```python
from build123d import *

# Parameters (mm, degrees)
SKETCH_1_W      = 5
SKETCH_1_H      = 60
EXTRUDE_1_DEPTH = 2
SKETCH_2_W      = 3
SKETCH_2_H      = 10
EXTRUDE_2_DEPTH = 10.5
SKETCH_3_W      = 15
SKETCH_3_H      = 60
EXTRUDE_3_DEPTH = 1.5


with BuildPart() as part:
    # 草图1 → 凸台-拉伸1 (new body)
    with BuildSketch(Plane(origin=(0, 0, 0), x_dir=(0, 0, -1), z_dir=(1, 0, 0))):
        with Locations((-1, 0)):
            Rectangle(SKETCH_1_W, SKETCH_1_H)
    extrude(amount=EXTRUDE_1_DEPTH)

    # 草图2 → 凸台-拉伸2 (add)
    with BuildSketch(Plane.ZY):
        with Locations((0, 20)):
            Rectangle(SKETCH_2_W, SKETCH_2_H)
        Rectangle(SKETCH_2_W, SKETCH_2_H)
        with Locations((0, -20)):
            Rectangle(SKETCH_2_W, SKETCH_2_H)
    extrude(amount=EXTRUDE_2_DEPTH)

    # 草图3 → 凸台-拉伸3 (add)
    with BuildSketch(Plane.ZY.offset(10.5)):
        Rectangle(SKETCH_3_W, SKETCH_3_H)
    extrude(amount=EXTRUDE_3_DEPTH)


solid = part.part
```
Check sheet for the modelled part. Datum: model origin and axes. Units: mm. A direction names the side the tool comes from. Round coordinates to 2 decimals unless told otherwise and drop trailing zeros. Loops run counter-clockwise (first coordinate to the right, second up) from the corner with the lowest first, then second, coordinate; pieces in that order, holes last. Notation, with made-up numbers: M -36,39 L 16,39 A29 cw 16,68 Z; hole C 87,-12.75 d10. An arc over 180 degrees is marked long. Answer as a JSON object with one key per item and string values.
1. Section check A-A (x = -3.5). Record the boundary of the cut face in (y, z), plus the area to 3 significant figures.
Reply:
{"outline": "M -25,-1.5 L -15,-1.5 L -15,1.5 L -25,1.5 Z; M -5,-1.5 L 5,-1.5 L 5,1.5 L -5,1.5 Z; M 15,-1.5 L 25,-1.5 L 25,1.5 L 15,1.5 Z", "area": "90.0 mm²"}
2. Scan lines: line 1 (Y direction, x = -10, z = 1); line 2 (X direction, y = 0, z = 2); line 3 (X direction, y = 3, z = -3.75). Record each from-to range of solid material in increasing order.
Reply:
{"line 1": "y = -25 to -15, -5 to 5, 15 to 25", "line 2": "x = -12 to -10.5, 0 to 2", "line 3": "x = -12 to -10.5"}
3. Access from +Z, -Z, +X, -X, +Y, -Y to the whole of each face (thin tool, end or side, straight path). Record for faces 5 (the flat face through (-5, -25, 0)), 6 (the flat face through (-5, 15, 0)), 7 (the flat face through (1, 0, 3.5)).
Reply:
{"face 5": "+Z, -Z, -Y", "face 6": "+Z, -Z", "face 7": "+Z, +X, +Y, -Y"}
4. Gauge pin test, flat ends, axial feed: P1, Ø6, axis at x = 0, y = 16, coming from the +Z side; P2, Ø4, axis at x = -8, y = -3.5, coming from the -Z side; P3, Ø1.5, axis at x = -6, z = 0, coming from the +Y side. Record the tip position at first contact, or that the pin passes through.
Reply:
{"P1": "stops at z = 3.5", "P2": "stops at z = -1.5", "P3": "stops at y = 25"}
5. Section check B-B (z = 2.25). Record the boundary of the cut face in (x, y).
Reply:
{"outline": "M -12,-30 L -10.5,-30 L -10.5,30 L -12,30 Z; M 0,-30 L 2,-30 L 2,30 L 0,30 Z"}
6. Section check C-C (y = -6.5). Record the boundary of the cut face in (x, z).
Reply:
{"outline": "M -12,-7.5 L -10.5,-7.5 L -10.5,7.5 L -12,7.5 Z; M 0,-1.5 L 2,-1.5 L 2,3.5 L 0,3.5 Z"}
7. Section check D-D (y = 19.5). Record the boundary of the cut face in (x, z), plus the area to 3 significant figures.
Reply:
{"outline": "M -12,-7.5 L -10.5,-7.5 L -10.5,-1.5 L 2,-1.5 L 2,3.5 L 0,3.5 L 0,1.5 L -10.5,1.5 L -10.5,7.5 L -12,7.5 Z", "area": "64.0 mm²"}
8. Mould release check, pull along X, two halves, no side actions. Record for faces 1 (the flat face through (2, 0, 1)), 2 (the flat face through (-5, 25, 0)), 3 (the flat face through (-11, 0, 7.5)), 4 (the flat face through (-12, 0, 0)): pulls with the +X half, pulls with the -X half, needs draft (parallel to the pull), parting line crosses it, or undercut.
Reply:
{"face 1": "pulls with the +X half", "face 2": "undercut", "face 3": "needs draft", "face 4": "pulls with the -X half"}
